```python
from build123d import *

# Parameters (mm, degrees)
BOSS_EXTRUDE1_DEPTH = 2
SKETCH2_W           = 20.5
SKETCH2_H           = 2
SKETCH2_W_2         = 13
SKETCH2_H_2         = 18
SKETCH2_H_3         = 17.5
BOSS_EXTRUDE2_DEPTH = 9
SKETCH3_W           = 5
SKETCH3_H           = 3
SKETCH3_W_2         = 8
BOSS_EXTRUDE4_DEPTH = 17.5
SKETCH6_W           = 7.5
SKETCH6_H           = 3
CUT_EXTRUDE1_DEPTH  = 2.5
CUT_EXTRUDE3_DEPTH  = 3
SKETCH11_W          = 15
SKETCH11_H          = 11
BOSS_EXTRUDE5_DEPTH = 1.75
SKETCH12_W          = 15
SKETCH12_H          = 11
BOSS_EXTRUDE6_DEPTH = 1.75
CUT_EXTRUDE4_DEPTH  = 2
SKETCH14_W          = 39.5
SKETCH14_H          = 11
BOSS_EXTRUDE7_DEPTH = 4.5
SKETCH16_W          = 30
SKETCH16_H          = 11
BOSS_EXTRUDE8_DEPTH = 2.5


with BuildPart() as part:
    # Sketch1 → Boss-Extrude1 (new body)
    with BuildSketch(Plane(origin=(0, 0, 0), x_dir=(1, 0, 0), z_dir=(0, 1, 0))):
        Polygon((0, 25.5), (24.5, 25.5), (24.5, 23.75), (39.5, 23.75), (39.5, 1.75), (24.5, 1.75), (24.5, 0), (0, 0), align=None)
    extrude(amount=BOSS_EXTRUDE1_DEPTH)

    # Sketch2 → Boss-Extrude2 (add)
    with BuildSketch(Plane(origin=(0, 2, 0), x_dir=(1, 0, 0), z_dir=(0, 1, 0))):
        Polygon((24.5, 23.75), (24.5, 25.5), (0, 25.5), (0, 0), (24.5, 0), (24.5, 1.75), (39.5, 1.75), (39.5, 23.75), align=None)
        with Locations((12.25, 22.5)):
            Rectangle(SKETCH2_W, SKETCH2_H, mode=Mode.SUBTRACT)
        with Locations((31, 12.75)):
            Rectangle(SKETCH2_W_2, SKETCH2_H_2, mode=Mode.SUBTRACT)
        with Locations((12.25, 10.75)):
            Rectangle(SKETCH2_W, SKETCH2_H_3, mode=Mode.SUBTRACT)
    extrude(amount=BOSS_EXTRUDE2_DEPTH)

    # Sketch3 → Boss-Extrude4 (add)
    with BuildSketch(Plane.XY.offset(-19.5)):
        with Locations((4.5, 3.5)):
            Rectangle(SKETCH3_W, SKETCH3_H)
        with Locations((18.5, 3.5)):
            Rectangle(SKETCH3_W_2, SKETCH3_H)
    extrude(amount=BOSS_EXTRUDE4_DEPTH)

    # Sketch6 → Cut-Extrude1 (cut)
    with BuildSketch(Plane.XY.offset(-19.5)):
        with Locations((10.75, 3.5)):
            Rectangle(SKETCH6_W, SKETCH6_H)
    extrude(amount=-CUT_EXTRUDE1_DEPTH, mode=Mode.SUBTRACT)

    # Sketch7 → Cut-Extrude3 (cut)
    with BuildSketch(Plane(origin=(0, 11, 0), x_dir=(1, 0, 0), z_dir=(0, 1, 0))):
        Polygon((24.5, 3.75), (22.5, 3.75), (22.5, 19.5), (2, 19.5), (2, 21.5), (22.5, 21.5), (22.5, 21.75), (24.5, 21.75), (24.5, 21.5), (24.5, 19.5), align=None)
    extrude(amount=-CUT_EXTRUDE3_DEPTH, mode=Mode.SUBTRACT)

    # Sketch11 → Boss-Extrude5 (add)
    with BuildSketch(Plane.XY.offset(-1.75)):
        with Locations((32, 5.5)):
            Rectangle(SKETCH11_W, SKETCH11_H)
    extrude(amount=BOSS_EXTRUDE5_DEPTH)

    # Sketch12 → Boss-Extrude6 (add)
    with BuildSketch(Plane(origin=(0, 0, -23.75), x_dir=(-1, 0, 0), z_dir=(0, 0, -1))):
        with Locations((-32, 5.5)):
            Rectangle(SKETCH12_W, SKETCH12_H)
    extrude(amount=BOSS_EXTRUDE6_DEPTH)

    # Sketch13 → Cut-Extrude4 (cut)
    with BuildSketch(Plane(origin=(2, 0, 0), x_dir=(0, 0, -1), z_dir=(1, 0, 0))):
        with BuildLine():
            Line((6.28, 7.5), (6.28, 8.21))
            ThreePointArc((6.28, 8.21), (6.646116524, 9.093883476), (7.53, 9.46))
            Line((7.53, 9.46), (13.97, 9.46))
            ThreePointArc((13.97, 9.46), (14.853883476, 9.093883476), (15.22, 8.21))
            Line((15.22, 8.21), (15.22, 7.5))
            ThreePointArc((15.22, 7.5), (14.853883476, 6.616116524), (13.97, 6.25))
            Line((13.97, 6.25), (7.53, 6.25))
            ThreePointArc((7.53, 6.25), (6.646116524, 6.616116524), (6.28, 7.5))
        make_face()
    extrude(amount=-CUT_EXTRUDE4_DEPTH, mode=Mode.SUBTRACT)

    # Sketch14 → Boss-Extrude7 (add)
    with BuildSketch(Plane.XY):
        with Locations((19.75, 5.5)):
            Rectangle(SKETCH14_W, SKETCH14_H)
    extrude(amount=BOSS_EXTRUDE7_DEPTH)

    # Sketch16 → Boss-Extrude8 (add)
    with BuildSketch(Plane(origin=(39.5, 0, 0), x_dir=(0, 0, -1), z_dir=(1, 0, 0))):
        with Locations((10.5, 5.5)):
            Rectangle(SKETCH16_W, SKETCH16_H)
    extrude(amount=BOSS_EXTRUDE8_DEPTH)


solid = part.part
```
For this review, take the finished solid that the model builds, in its own axes (mm). A direction names the side the tool comes from. Give positions to 0.01 mm unless a question says otherwise; leave off trailing zeros. Write each loop counter-clockwise with the first axis right and the second up, starting at its lowest first coordinate (ties: lowest second). Pieces come first, ordered by that corner, then holes.
Item 1: Insertion check: P1, Ø4, axis at x = 5, z = -12, coming from the +Y side; P2, Ø2, axis at x = 8.5, z = -8, coming from the +Y side. Each pin has a flat end and moves straight along its axis. Give the tip position at first contact, or say it passes through.
Item 2: Take a section at D-D (x = 17.5). Give the boundary of the cut face in (y, z), and give its area (3 significant figures).
Item 3: Take a section at C-C (y = 3.25). Give the boundary of the cut face in (x, z), and give its area (3 significant figures).
Item 4: Wall thickness on probe 1 along X at (y, z) = (7, -17.5); probe 2 along X at (y, z) = (2.75, -9.5); probe 3 along Z at (x, y) = (6, 5.75): over which ranges is each line inside the solid? List them lowest first.
Item 5: The part is to be moulded in two halves that separate along X. For faces 4 (the face through (12, 6, -19.5)), 5 (the face through (10, 2, -15)), 6 (the face through (0, 5, -11)), 7 (the face through (25, 11, 0)), say which applies: +X half, -X half, draft (parallel to the pull), parting line (faces both ways), or undercut.
Item 6: Machinability: for faces 1 (the face through (1.014, 6.626, -14.864)), 2 (the face through (2, 6, -15)), 3 (the face through (11, 5, -20)), which of the approach directions +Z, -Z, +X, -X, +Y, -Y give a long, thin tool a straight path to every point of the face, cutting with its end or side? Answer none if there is none.
Item 7: Take a section at B-B (z = -10). Give the boundary of the cut face in (x, y).
Item 8: Take a section at A-A (x = 8). Give the boundary of the cut face in (y, z), and give its area (4 significant figures).
Established:
1. P1: stops at y = 5
1. P2: stops at y = 2
2. outline: (0, -25.5) - (11, -25.5) - (11, -23.5) - (2, -23.5) - (2, -21.5) - (8, -21.5) - (8, -19.5) - (5, -19.5) - (5, -2) - (11, -2) - (11, 4.5) - (0, 4.5) - close
2. area: 201 mm2
3. outline: (0, -25.5) - (42, -25.5) - (42, 4.5) - (0, 4.5) - close; hole (2, -23.5) - (22.5, -23.5) - (22.5, -21.5) - (14.5, -21.5) - (14.5, -2) - (7, -2) - (7, -21.5) - (2, -21.5) - close; hole (24.5, -21.75) - (37.5, -21.75) - (37.5, -3.75) - (24.5, -3.75) - close
3. area: 839 mm2
4. probe 1: x = 0 to 2, 22.5 to 24.5, 37.5 to 42
4. probe 2: x = 0 to 7, 14.5 to 24.5, 37.5 to 42
4. probe 3: z = -25.5 to -23.5, -21.5 to -19.5, -2 to 4.5
5. face 4: undercut
5. face 5: undercut
5. face 6: -X half
5. face 7: draft
6. face 1: -X
6. face 2: +Y
6. face 3: none
7. outline: (0, 0) - (42, 0) - (42, 11) - (37.5, 11) - (37.5, 2) - (24.5, 2) - (24.5, 8) - (22.5, 8) - (22.5, 5) - (14.5, 5) - (14.5, 2) - (7, 2) - (7, 5) - (2, 5) - (2, 6.25) - (0, 6.25) - close; (0, 9.46) - (2, 9.46) - (2, 11) - (0, 11) - close
8. outline: (0, -25.5) - (11, -25.5) - (11, -23.5) - (2, -23.5) - (2, -2) - (11, -2) - (11, 4.5) - (0, 4.5) - close; (5, -21.5) - (8, -21.5) - (8, -19.5) - (5, -19.5) - close
8. area: 142.5 mm2
